Input: part model. Units: mm. Frame: model coordinates. Face numbers are marked on the shaded views. A direction names the side the tool comes from. Give positions to 0.01 mm unless a question says otherwise; leave off trailing zeros. Write each loop counter-clockwise with the first axis right and the second up, starting at its lowest first coordinate (ties: lowest second). Pieces come first, ordered by that corner, then holes. Notation, with made-up numbers: (11, -4) -> (48, -4) arc R20 cw to (48, 33) -> close; hole circle Ø1 at (86, -29.5). An arc over 180 degrees is marked (long way). Return JSON: item names as keys, results as strings. Group by question number.
Item 1: Section D-D, the plane z = 3. Count the separate pieces of the cut face and the enclosed holes in it, then the cut area to 3 significant figures.
Item 2: Mould query, pull axis X, two halves, no side actions, for the marked faces 6, 7 and 8. Classes: released by +X, released by -X, zero draft, split by the parting line, or undercut.
Item 3: Pin query (flat end, axial travel): P1, Ø0.6, axis at y = 5.5, z = 3, coming from the -X side; P2, Ø2, axis at x = 1.5, z = 2.5, coming from the -Y side; P3, Ø1, axis at y = -6, z = 3, coming from the -X side; P4, Ø1.6, axis at y = -6.5, z = 2.5, coming from the +X side. Return the tip coordinate at first contact, or that it passes through.
Item 4: Section A-A, the plane y = -2.6. Return loops of the section in (x, z) (3 decimals).
Item 5: Section C-C, the plane x = 4.75. Return loops of the section in (y, z) (3 decimals), then the cut area to 3 significant figures.
Item 6: Section B-B, the plane x = -0.25. Return loops of the section in (y, z).
Item 7: Set-up query: the marked faces 1, 2, 3, 4 and 5. Return all of +Z, -Z, +X, -X, +Y, -Y with unobstructed straight access to the full face (end or side cutting, diameter ignored); none if empty.
Item 8: Line query: line 1 (X direction, y = -7, z = 4); line 2 (Y direction, x = -4.75, z = 5) (3 decimals); line 3 (Y direction, x = 4.75, z = 4.5) (3 decimals). Output: solid intervals per line, ascending. Write a range as [from, to].
from build123d import *

# Parameters (mm, degrees)
SKETCH_1_W               = 19.8
SKETCH_1_H               = 10.2
EXTRUDE_1_DEPTH          = 6.4
CUT_EXTRUDE_1_DEPTH      = 13.844454056
CUT_EXTRUDE_1_DEPTH_BACK = 13.844454056
SKETCH_3_R               = 1.175
CUT_EXTRUDE_2_DEPTH      = 13.844454056
SKETCH_4_W               = 2
SKETCH_4_H               = 3.7
EXTRUDE_2_DEPTH          = 0.9
FILLET_2_R               = 0.5
FILLET_3_R               = 1
SKETCH_6_W               = 0.5
SKETCH_6_H               = 3.2
EXTRUDE_3_DEPTH          = 3.9
CHAMFER_1_SIZE           = 0.5
EXTRUDE_4_DEPTH          = 2


with BuildPart() as part:
    # 草图1 → 凸台-拉伸1 (new body)
    with BuildSketch(Plane.XY):
        Rectangle(SKETCH_1_W, SKETCH_1_H)
    extrude(amount=EXTRUDE_1_DEPTH)

    # 草图2 → 切除-拉伸1 (cut, two sides: drawn at the far end of the back side and taken through both)
    with BuildSketch(Plane.XY.offset(6.4).offset(-CUT_EXTRUDE_1_DEPTH_BACK)):
        Polygon((9.9, 5.1), (0.905266145, 5.1), (1.605266145, 4.4), (9.9, 4.4), align=None)
    extrude(amount=CUT_EXTRUDE_1_DEPTH + CUT_EXTRUDE_1_DEPTH_BACK, mode=Mode.SUBTRACT)

    # 草图3 → 切除-拉伸2 (cut, through all)
    with BuildSketch(Plane.XY.offset(6.4)):
        with Locations((-4.75, -2.6)):
            Circle(SKETCH_3_R)
        with Locations((4.75, -2.6)):
            Circle(SKETCH_3_R)
    extrude(amount=-CUT_EXTRUDE_2_DEPTH, mode=Mode.SUBTRACT)

    # 草图4 → 凸台-拉伸2 (add)
    with BuildSketch(Plane(origin=(0, 5.1, 0), x_dir=(1, 0, 0), z_dir=(0, 1, 0))):
        with Locations((-2.85, -3.2)):
            Rectangle(SKETCH_4_W, SKETCH_4_H)
    extrude(amount=EXTRUDE_2_DEPTH)

    # 圆角2
    fillet_2_edges = [part.edges().sort_by_distance(p)[0] for p in [
        (9.9, 4.4, 3.2),
        (-9.9, 5.1, 3.2),
        (9.9, -5.1, 3.2),
        (-9.9, -5.1, 3.2),
    ]]
    fillet(fillet_2_edges, radius=FILLET_2_R)

    # 圆角3
    # the kernel refuses this fillet: 1 mm, written as the material it takes off along each edge
    with BuildSketch(Plane(origin=(-1.85, 6, -1.137468593), x_dir=(0, -1, 0), z_dir=(0, 0, 1)), Plane(origin=(-3.85, 6, 7.537468593), x_dir=(0, -1, 0), z_dir=(0, 0, -1))) as fillet_3_piece_1:
        with BuildLine():
            CenterArc((1, -0.994987437), FILLET_3_R, 95.739170477, 84.260829523)
            Line((0, -0.994987437), (-0.02, -0.994987437))
            Line((-0.02, -0.994987437), (-0.02, 0))
            Line((-0.02, 0), (0, 0.02))
            ThreePointArc((0, 0.02), (0.45, 0.02), (0.898, 0.019899749))
            Line((0.898, 0.019899749), (0.9, 0))
        make_face()
    extrude(amount=8.674937186, mode=Mode.SUBTRACT)

    # 草图6 → 凸台-拉伸3 (add)
    with BuildSketch(Plane.XZ.offset(5.1)):
        with Locations((-8.05, 3.2)):
            Rectangle(SKETCH_6_W, SKETCH_6_H)
        with Locations((0.75, 3.2)):
            Rectangle(SKETCH_6_W, SKETCH_6_H)
        with Locations((8.05, 3.2)):
            Rectangle(SKETCH_6_W, SKETCH_6_H)
    extrude(amount=EXTRUDE_3_DEPTH)

    # 倒角1
    chamfer_1_edges = [part.edges().sort_by_distance(p)[0] for p in [
        (0.75, -9, 4.8),
        (0.75, -9, 1.6),
        (8.05, -9, 4.8),
        (8.05, -9, 1.6),
        (-8.05, -9, 4.8),
        (-8.05, -9, 1.6),
    ]]
    chamfer(chamfer_1_edges, length=CHAMFER_1_SIZE)

    # 草图7 → 凸台-拉伸4 (add, symmetric)
    with BuildSketch(Plane(origin=(0, 0, 3.2), x_dir=(-1, 0, 0), z_dir=(0, 0, -1))):
        Polygon((4.9, 5.1), (4.9, 6.3), (-9.25, 6.3), (-9.25, 5.8), (4.4, 5.8), (4.4, 5.1), align=None)
    extrude(amount=EXTRUDE_4_DEPTH, both=True)


solid = part.part
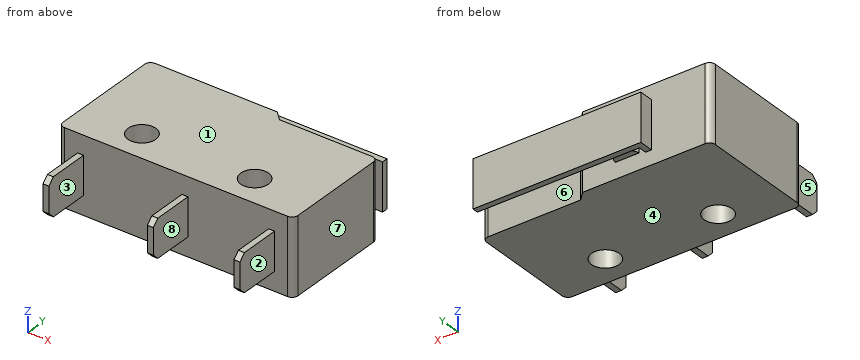
Answer below:
{
 "1": {"separate pieces": "1", "enclosed holes": "3", "area": "202 mm2"},
 "2": {"face 6": "zero draft", "face 7": "released by +X", "face 8": "undercut"},
 "3": {"P1": "stops at x = -4.9", "P2": "stops at y = -9", "P3": "stops at x = -8.3", "P4": "stops at x = 8.3"},
 "4": {"outline": "(-9.9, 0) -> (-5.925, 0) -> (-5.925, 6.4) -> (-9.9, 6.4) -> close; (-3.575, 0) -> (3.575, 0) -> (3.575, 6.4) -> (-3.575, 6.4) -> close; (5.925, 0) -> (9.9, 0) -> (9.9, 6.4) -> (5.925, 6.4) -> close"},
 "5": {"outline": "(-5.1, 0) -> (-3.775, 0) -> (-3.775, 6.4) -> (-5.1, 6.4) -> close; (-1.425, 0) -> (4.4, 0) -> (4.4, 6.4) -> (-1.425, 6.4) -> close; (5.8, 1.2) -> (6.3, 1.2) -> (6.3, 5.2) -> (5.8, 5.2) -> close", "area": "47.8 mm2"},
 "6": {"outline": "(-5.1, 0) -> (5.1, 0) -> (5.1, 6.4) -> (-5.1, 6.4) -> close; (5.8, 1.2) -> (6.3, 1.2) -> (6.3, 5.2) -> (5.8, 5.2) -> close"},
 "7": {"face 1": "+Z, +X, -X, +Y, -Y", "face 2": "+Z, -Z, +X, -Y", "face 3": "+Z, -Z, -Y", "face 4": "-Z, +X, -X, +Y, -Y", "face 5": "+Z, -Z, -X, -Y"},
 "8": {"line 1": "x = [-8.3, -7.8], [0.5, 1], [7.8, 8.3]", "line 2": "y = [-5.1, -3.775], [-1.425, 6.3]", "line 3": "y = [-5.1, -3.775], [-1.425, 4.4], [5.8, 6.3]"}
}
